Could you check a few things on this model? Use its own coordinates, in mm. A direction names the side the tool comes from. Coordinates: 2 decimals unless noted, no trailing zeros. Loops run counter-clockwise (first coordinate to the right, second up) from the corner with the lowest first, then second, coordinate; pieces in that order, holes last.
Autodesk Inventor part; units mm, degrees
ref_plane "YZ Plane" through (0, 0, 0) normal (1, 0, 0) x (0, 1, 0)
ref_plane "XZ Plane" through (0, 0, 0) normal (0, 1, 0) x (-1, 0, 0)
ref_plane "XY Plane" through (0, 0, 0) normal (0, 0, 1) x (1, 0, 0)
sketch "Sketch1" plane through (0, 0, 0) normal (0, 1, 0) x (-1, 0, 0)
  line L0 (0, 0) -> (-100, 0)
  line L1 (-100, 0) -> (-100, -100)
  line L2 (-100, -100) -> (0, -100)
  line L3 (0, -100) -> (0, 0)
  dimension "d0" = 100
  dimension "d1" = 100
extrude "Extrusion1" add sketch "Sketch1" along normal blind 1000
sketch "Sketch2" plane through (0, 1000, 0) normal (0, 1, 0) x (1, 0, 0)
  line L0 (100, 0) -> (100, 100)
  line L1 (100, 100) -> (0, 100)
  circle A0 centre (50, 50) radius 10
  circle A1 centre (50, 50) radius 40
  point P0 (0, 0)
  dimension "d4" = 20
  dimension "d5" = 80
extrude "Extrusion2" cut sketch "Sketch2" against normal blind 175 contours A0
extrude "Extrusion3" add sketch "Sketch2" along normal blind 5
fillet "Fillet1" radius 10 1 edges at (10, 1005, -50)
fillet "Fillet2" radius 10 4 edges at (100, 500, 0) (0, 500, 0) (0, 500, -100) (100, 500, -100)
properties part number "pneumatic_cylinder_ body" material "Stainless Steel"
(1) Imagine slicing it at A-A, the plane z = -50. Write out the boundary of the cut face in (x, y).
Answers:
outline: (0, 0) - (100, 0) - (100, 1000) - (90, 1000) arc R10 ccw to (81.34, 1005) - (60, 1005) - (60, 825) - (40, 825) - (40, 1005) - (18.66, 1005) arc R10 ccw to (10, 1000) - (0, 1000) - close
(2) Imagine slicing it at B-B, the plane x = 50. Write out the boundary of the cut face in (y, z), and give its area (3 significant figures).
Answers:
outline: (0, -100) - (1000, -100) - (1000, -90) arc R10 ccw to (1005, -81.34) - (1005, -60) - (825, -60) - (825, -40) - (1005, -40) - (1005, -18.66) arc R10 ccw to (1000, -10) - (1000, 0) - (0, 0) - close
area: 96,800 mm2
(3) We'd pull the mould along Z, two halves only. Please class faces 1 (the face through (50, 825, -50)), 2 (the face through (49, 493, 0)), 3 (the face through (100, 493, -49)), 4 (the face through (42, 914, -56)): +Z half, -Z half, draft (parallel to the pull), parting line (faces both ways), or undercut.
Answers:
face 1: undercut
face 2: +Z half
face 3: draft
face 4: undercut
(4) Which directions (+Z, -Z, +X, -X, +Y, -Y) give clear straight access to the entire face, cutting with the end or side of a thin tool? Please do faces 5 (the face through (51, 493, -100)), 6 (the face through (84, 1000, -27)).
Answers:
face 5: -Z, +X, -X, +Y, -Y
face 6: +Y
(5) For pin 1 (12 mm diameter, centred on y = 235, z = -71.5, fed in from -X), with a flat end and sliding along its axis, tell me the tip position at first contact or that it passes through.
Answers:
pin 1: stops at x = 0
(6) I need wall thicknesses on probe 1 along Z at (x, y) = (50, 896.5); probe 2 along X at (y, z) = (909, -50); probe 3 along Y at (x, z) = (14, -69.5). Which ranges of each line are inside material? Lowest first, please.
Answers:
probe 1: z = -100 to -60, -40 to 0
probe 2: x = 0 to 40, 60 to 100
probe 3: y = 0 to 1000
